from build123d import *

# Parameters (mm, degrees)
BOSS_EXTRUDE1_DEPTH = 6.35


with BuildPart() as part:
    # Sketch1 → Boss-Extrude1 (new body)
    with BuildSketch(Plane.XY):
        with BuildLine():
            Line((-16.886131477, 10.741733319), (-15.875, 11.590173369))
            Line((-15.875, 11.590173369), (-15.875, 19.879509656))
            Line((-15.875, 19.879509656), (-33.221751492, 5.323856877))
            Line((-33.221751492, 5.323856877), (-36.396751492, 10.823118191))
            ThreePointArc((-36.396751492, 10.823118191), (-39.371085636, 9.639070453), (-41.418515119, 7.178041166))
            Line((-41.418515119, 7.178041166), (-41.418515119, -4.201143123))
            Line((-41.418515119, -4.201143123), (-34.925, -4.201143123))
            Line((-34.925, -4.201143123), (-34.925, 2.148856877))
            Line((-34.925, 2.148856877), (-28.575, 2.148856877))
            Line((-28.575, 2.148856877), (-28.575, -4.201143123))
            Line((-28.575, -4.201143123), (-22.225, -4.201143123))
            Line((-22.225, -4.201143123), (-22.225, 2.148856877))
            Line((-22.225, 2.148856877), (-15.875, 2.148856877))
            Line((-15.875, 2.148856877), (-15.875, -4.201143123))
            Line((-15.875, -4.201143123), (-9.525, -4.201143123))
            Line((-9.525, -4.201143123), (-9.525, 2.148856877))
            Line((-9.525, 2.148856877), (9.525, 2.148856877))
            Line((9.525, 2.148856877), (9.525, -4.201143123))
            Line((9.525, -4.201143123), (15.875, -4.201143123))
            Line((15.875, -4.201143123), (15.875, 2.148856877))
            Line((15.875, 2.148856877), (22.225, 2.148856877))
            Line((22.225, 2.148856877), (22.225, -4.201143123))
            Line((22.225, -4.201143123), (28.575, -4.201143123))
            Line((28.575, -4.201143123), (28.575, 2.148856877))
            Line((28.575, 2.148856877), (34.925, 2.148856877))
            Line((34.925, 2.148856877), (34.925, -4.201143123))
            Line((34.925, -4.201143123), (41.418515119, -4.201143123))
            Line((41.418515119, -4.201143123), (41.418515119, 7.178041166))
            ThreePointArc((41.418515119, 7.178041166), (39.371085636, 9.639070453), (36.396751492, 10.823118191))
            Line((36.396751492, 10.823118191), (33.221751492, 5.323856877))
            Line((33.221751492, 5.323856877), (15.875, 19.879509656))
            Line((15.875, 19.879509656), (15.875, 11.590173369))
            Line((15.875, 11.590173369), (16.886131477, 10.741733319))
            ThreePointArc((16.886131477, 10.741733319), (17.263200841, 9.334491295), (16.069791213, 8.498856877))
            Line((16.069791213, 8.498856877), (3.175, 8.498856877))
            Line((3.175, 8.498856877), (3.175, 22.246738685))
            Line((3.175, 22.246738685), (9.525, 16.918456027))
            Line((9.525, 16.918456027), (9.525, 25.207792314))
            Line((9.525, 25.207792314), (6.122551982, 28.062785191))
            ThreePointArc((6.122551982, 28.062785191), (0, 30.29121187), (-6.122551982, 28.062785191))
            Line((-6.122551982, 28.062785191), (-9.525, 25.207792314))
            Line((-9.525, 25.207792314), (-9.525, 16.918456027))
            Line((-9.525, 16.918456027), (-3.175, 22.246738685))
            Line((-3.175, 22.246738685), (-3.175, 8.498856877))
            Line((-3.175, 8.498856877), (-16.069791213, 8.498856877))
            ThreePointArc((-16.069791213, 8.498856877), (-17.263200841, 9.334491295), (-16.886131477, 10.741733319))
        make_face()
    extrude(amount=BOSS_EXTRUDE1_DEPTH)


solid = part.part
Geometry: final body of the model. Coordinates: model frame, mm. A direction names the side the tool comes from. Give positions to 0.01 mm unless a question says otherwise; leave off trailing zeros. Write each loop counter-clockwise with the first axis right and the second up, starting at its lowest first coordinate (ties: lowest second). Pieces come first, ordered by that corner, then holes. Notation, with made-up numbers: M 35,77.25 L 39,77.25 A18 cw 39,106.25 Z; hole C 49,-14 d3. An arc over 180 degrees is marked long. Answer in a Markdown table with one row per item. Add a question column.
(1) Mould query, pull axis X, two halves, no side actions, for faces 1 (the flat face through (25, -4.201, 3)), 2 (the flat face through (41.419, 1, 3)), 3 (the cylindrical face through (-39.33, 9.67, 3.13)), 4 (the flat face through (34.925, -1, 3)). Classes: +X half, -X half, draft (parallel to the pull), parting line (faces both ways), or undercut.
(2) Section D-D on y = 23.5. Return loops of the section in (x, z) (3 decimals).
(3) Section B-B on y = 9.5. Return loops of the section in (x, z) (3 decimals).
(4) Ray query, line 1 (X direction, y = -3, z = 1.25) (3 decimals); line 2 (X direction, y = 11, z = 1.5) (3 decimals); line 3 (X direction, y = 8, z = 3). Return the intervals inside material, ascending.
(5) Reachability of faces 5 (the flat face through (-9.525, 21, 3)), 6 (the flat face through (-9.525, -1, 3)), 7 (the flat face through (-1, 9, 0)), 8 (the cylindrical face through (-17.256, 9.314, 3.131)) from +Z, -Z, +X, -X, +Y, -Y: full face, straight path, thin tool, end or side. Return the list, or none.
(6) Section C-C on x = 4. Return loops of the section in (y, z), and give its area (3 significant figures).
(7) Section A-A on y = 16. Return loops of the section in (x, z) (3 decimals), and give its area (3 significant figures).
(8) First-contact query: pin 1 (1.9 mm diameter, centred on x = 19, z = 4, fed in from -Y); pin 2 (3 mm diameter, centred on y = 14.5, z = 4, fed in from -X); pin 3 (2 mm diameter, centred on x = -22, y = 10.5, fed in from -Z); pin 4 (3 mm diameter, centred on y = 22.5, z = 4, fed in from -X) (3 decimals). Flat tips, straight axial feed; report the tip coordinate or a pass-through.
Result set:
| question | item | result |
|---|---|---|
| 1 | face 1 | draft |
| 1 | face 2 | +X half |
| 1 | face 3 | -X half |
| 1 | face 4 | undercut |
| 2 | outline | M -9.525,0 L 9.525,0 L 9.525,6.35 L -9.525,6.35 Z |
| 3 | outline | M -39.556,0 L -35.633,0 L -35.633,6.35 L -39.556,6.35 Z; M -28.245,0 L -17.311,0 L -17.311,6.35 L -28.245,6.35 Z; M -3.175,0 L 3.175,0 L 3.175,6.35 L -3.175,6.35 Z; M 17.311,0 L 28.245,0 L 28.245,6.35 L 17.311,6.35 Z; M 35.633,0 L 39.556,0 L 39.556,6.35 L 35.633,6.35 Z |
| 4 | line 1 | x = -41.419 to -34.925, -28.575 to -22.225, -15.875 to -9.525, 9.525 to 15.875, 22.225 to 28.575, 34.925 to 41.419 |
| 4 | line 2 | x = -26.457 to -16.578, -3.175 to 3.175, 16.578 to 26.457 |
| 4 | line 3 | x = -40.95 to -34.77, -30.03 to 30.03, 34.77 to 40.95 |
| 5 | face 5 | +Z, -Z, +Y |
| 5 | face 6 | +Z, -Z, -Y |
| 5 | face 7 | -Z, +X, -X, +Y, -Y |
| 5 | face 8 | +Z, -Z |
| 6 | outline | M 2.15,0 L 8.5,0 L 8.5,6.35 L 2.15,6.35 Z; M 21.55,0 L 29.41,0 L 29.41,6.35 L 21.55,6.35 Z |
| 6 | area | 90.2 mm^2 |
| 7 | outline | M -20.498,0 L -15.875,0 L -15.875,6.35 L -20.498,6.35 Z; M -3.175,0 L 3.175,0 L 3.175,6.35 L -3.175,6.35 Z; M 15.875,0 L 20.498,0 L 20.498,6.35 L 15.875,6.35 Z |
| 7 | area | 99.0 mm^2 |
| 8 | pin 1 | stops at y = 2.15 |
| 8 | pin 2 | stops at x = -24.07 |
| 8 | pin 3 | stops at z = 0 |
| 8 | pin 4 | stops at x = -9.525 |
